```python
from build123d import *

# Parameters (mm, degrees)
F1_DEPTH = 25.4
F3_DEPTH = 25.4
F4_R     = 5.08


with BuildPart() as f1:
    # F0 (on Front) → F1 (new body)
    with BuildSketch(Plane.XZ):
        Polygon((-45.568943, 31.75), (-45.065421, 0), (11.581057, 0), (11.581057, 31.75), align=None)
    extrude(amount=F1_DEPTH)

    # F2 (on face) → F3 (cut)
    with BuildSketch(Plane.XZ.offset(25.4)):
        with BuildLine():
            Line((11.581057, 31.75), (-13.818943, 31.75))
            ThreePointArc((-13.818943, 31.75), (-2.817404, 22.003079), (11.581057, 19.05))
            Line((11.581057, 19.05), (11.581057, 31.75))
        make_face()
    extrude(amount=-F3_DEPTH, mode=Mode.SUBTRACT)

    # F4
    f4_edges = [f1.edges().sort_by_distance(p)[0] for p in [
        (-45.568943, -12.7, 31.75),
    ]]
    fillet(f4_edges, radius=F4_R)


solid = f1.part
```
Check sheet for the modelled part. Datum: model origin and axes. Units: mm. Coordinates: 2 decimals unless noted, no trailing zeros. Loops run counter-clockwise (first coordinate to the right, second up) from the corner with the lowest first, then second, coordinate; pieces in that order, holes last. Notation, with made-up numbers: M -2.75,-9.5 L 26.25,-9.5 A23 cw 26.25,7.5 Z; hole C 87.25,-32 d7. An arc over 180 degrees is marked long. Answer as a JSON object with one key per item and string values.
1. Sectioned sample at B-B on x = -6. Record the cut outline in (y, z).
Outcome:
{"outline": "M -25.4,0 L 0,0 L 0,23.86 L -25.4,23.86 Z"}
2. Sectioned sample at C-C on z = 30.5. Record the cut outline in (x, y).
Outcome:
{"outline": "M -43.75,-25.4 L -12.94,-25.4 L -12.94,0 L -43.75,0 Z"}
3. Sectioned sample at A-A on y = -21.25. Record the cut outline in (x, z), and give its area (3 significant figures).
Outcome:
{"outline": "M -45.49,26.59 L -45.07,0 L 11.58,0 L 11.58,19.05 A28.44 cw -13.82,31.75 L -40.41,31.75 A5.08 ccw Z", "area": "1,570 mm²"}
4. Depth check by flat-ended pin: P1, Ø2, axis at y = -8, z = 19.5, coming from the -X side; P2, Ø8, axis at y = -7, z = 5.5, coming from the -X side; P3, Ø8, axis at x = -8.5, y = -14, coming from the +Z side. Enter the tip coordinate at first touch or a pass-through.
Outcome:
{"P1": "x = -45.39", "P2": "x = -45.22", "P3": "z = 29.92"}
5. Scan lines: L1, parallel to Z at x = -10, y = -6.75; L2, parallel to Z at x = 6, y = -7.25; L3, parallel to X at y = -3.5, z = 25. Record each from-to range of solid material in increasing order. Write a range as from..to.
Outcome:
{"L1": "0..27.12", "L2": "0..19.27", "L3": "-45.46..-7.57"}
